from build123d import *

# Parameters (mm, degrees)
EXTRUDE_1_DEPTH          = 24
CUT_EXTRUDE_2_DEPTH      = 54.111509792
CUT_EXTRUDE_2_DEPTH_BACK = 40
CUT_EXTRUDE_START        = -40
CUT_EXTRUDE_3_DEPTH      = 40
SKETCH_8_R               = 2
SKETCH_8_R_2             = 5
CUT_EXTRUDE_4_DEPTH      = 40
SKETCH_9_R               = 1.5
CUT_EXTRUDE_5_DEPTH      = 10


with BuildPart() as part:
    # 草图1 → 凸台-拉伸1 (new body)
    with BuildSketch(Plane.XY):
        with BuildLine():
            Line((30, -7), (30, -34))
            Line((30, -34), (32.997461605, -34))
            Line((32.997461605, -34), (32.997461605, -3))
            ThreePointArc((32.997461605, -3), (32.118781948, -0.878679656), (29.997461605, 0))
            Line((29.997461605, 0), (0, 0))
            Line((0, 0), (0, -4))
            Line((0, -4), (27, -4))
            ThreePointArc((27, -4), (29.121320344, -4.878679656), (30, -7))
        make_face()
    extrude(amount=EXTRUDE_1_DEPTH)

    # 草图4 → 切除-拉伸2 (cut, two sides: drawn at the far end of the back side and taken through both)
    with BuildSketch(Plane(origin=(32.997461605, 0, 0), x_dir=(0, 0, -1), z_dir=(1, 0, 0)).offset(-CUT_EXTRUDE_2_DEPTH_BACK)):
        with BuildLine():
            Line((-24, -34), (-12, -34))
            ThreePointArc((-12, -34), (-20.485281374, -30.485281374), (-24, -22))
            Line((-24, -22), (-24, -34))
        make_face()
    extrude(amount=CUT_EXTRUDE_2_DEPTH + CUT_EXTRUDE_2_DEPTH_BACK, mode=Mode.SUBTRACT)

    # 草图7 → 切除-拉伸3 (cut)
    with BuildSketch(Plane(origin=(32.997461605, 0, 0), x_dir=(0, 0, -1), z_dir=(1, 0, 0)).offset(CUT_EXTRUDE_START)):
        with BuildLine():
            Line((0, -34), (0, -22))
            ThreePointArc((0, -22), (-3.514718626, -30.485281374), (-12, -34))
            Line((-12, -34), (0, -34))
        make_face()
    extrude(amount=CUT_EXTRUDE_3_DEPTH, mode=Mode.SUBTRACT)

    # 草图8 → 切除-拉伸4 (cut)
    with BuildSketch(Plane(origin=(0, 0, 0), x_dir=(1, 0, 0), z_dir=(0, 1, 0))):
        with Locations(Location((7.95757976, -5.000064267, 0), (0, 0, 270))):
            Circle(SKETCH_8_R)
        with Locations(Location((22, -19, 0), (0, 0, 270))):
            Circle(SKETCH_8_R)
        with Locations(Location((21.95757976, -5.000064267, 0), (0, 0, 270))):
            Circle(SKETCH_8_R)
        with Locations(Location((15, -12, 0), (0, 0, 270))):
            Circle(SKETCH_8_R_2)
        with Locations(Location((8, -19, 0), (0, 0, 270))):
            Circle(SKETCH_8_R)
    extrude(amount=-CUT_EXTRUDE_4_DEPTH, mode=Mode.SUBTRACT)

    # 草图9 → 切除-拉伸5 (cut)
    with BuildSketch(Plane(origin=(32.997461605, 0, 0), x_dir=(0, 0, -1), z_dir=(1, 0, 0))):
        with Locations((-12.027919591, -22.255700116)):
            Circle(SKETCH_9_R)
    extrude(amount=-CUT_EXTRUDE_5_DEPTH, mode=Mode.SUBTRACT)


solid = part.part
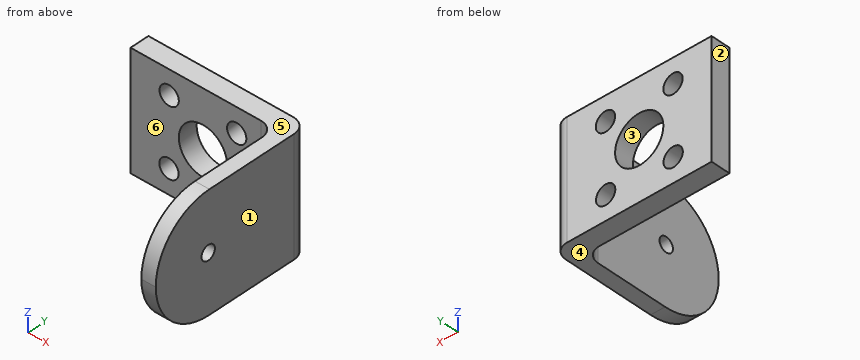
Work out the finished part from the listing and answer in its coordinate system (mm). Face numbers are marked on the shaded views. A direction names the side the tool comes from. Coordinates: 2 decimals unless noted, no trailing zeros. Loops run counter-clockwise (first coordinate to the right, second up) from the corner with the lowest first, then second, coordinate; pieces in that order, holes last. Notation, with made-up numbers: (53, -37) -> (72, -37) arc R24 ccw to (72, -14) -> close; hole circle Ø3 at (3, 6.25). An arc over 180 degrees is marked (long way). Write each question's results on one line, items separated by ' | '. Start each with the question number.
1) For the marked faces 5 and 6, determine the directions among +Z, -Z, +X, -X, +Y, -Y from which every point of the face is accessible in a straight line to the end or side of a thin tool.
2) Consider line 1 along X through (y, z) = (-1.3, 19); line 2 along Y through (x, z) = (27, 3); line 3 along X through (y, z) = (-29, 12). Determine where each line is inside the solid, lowest interval first.
3) The mould has two halves that part along X. Classify the marked faces 1, 2, 3 and 4: pulls with the +X half, pulls with the -X half, needs draft (parallel to the pull), parting line crosses it, or undercut.
4) Find section D-D on z = 22. Determine the outline of the cut face in (x, y).
5) Flat-ended cylindrical pins translate along their axes: P1, Ø2.5, axis at x = 8, z = 19, coming from the +Y side; P2, Ø12, axis at y = -19.5, z = 17, coming from the -X side; P3, Ø6.5, axis at x = 22, z = 19, coming from the -Y side; P4, Ø3, axis at y = -6.5, z = 8.5, coming from the -X side. Find the tip coordinate at first contact, or state that the pin passes through.
6) Find section C-C on y = -1.5. Determine the outline of the cut face in (x, z).
7) Find section A-A on z = 19. Determine the outline of the cut face in (x, y), then the cut area to 3 significant figures.
8) Find section B-B on x = 20.5. Determine the outline of the cut face in (y, z).
Response values:
1) face 5: +Z, +X, -X, +Y, -Y | face 6: +Z, -Z, -X, -Y
2) line 1: x = 0 to 6, 10 to 20, 24 to 32.47 | line 2: y = -4 to 0 | line 3: x = 30 to 33
3) face 1: pulls with the +X half | face 2: pulls with the -X half | face 3: undercut | face 4: needs draft
4) outline: (0, -4) -> (27, -4) arc R3 cw to (30, -7) -> (30, -28.63) -> (33, -28.63) -> (33, -3) arc R3 ccw to (30, 0) -> (0, 0) -> close
5) P1: passes through | P2: stops at x = 30 | P3: stops at y = -4 | P4: stops at x = 29.24
6) outline: (0, 0) -> (32.6, 0) -> (32.6, 24) -> (0, 24) -> close; hole circle Ø4 at (7.96, 5); hole circle Ø4 at (8, 19); hole circle Ø10 at (15, 12); hole circle Ø4 at (21.96, 5); hole circle Ø4 at (22, 19)
7) outline: (0, -4) -> (6, -4) -> (6, 0) -> (0, 0) -> close; (10, -4) -> (20, -4) -> (20, 0) -> (10, 0) -> close; (24, -4) -> (27, -4) arc R3 cw to (30, -7) -> (30, -31.75) -> (33, -31.75) -> (33, -3) arc R3 ccw to (30, 0) -> (24, 0) -> close | area: 183 mm^2
8) outline: (-4, 0) -> (0, 0) -> (0, 3.63) -> (-4, 3.63) -> close; (-4, 6.37) -> (0, 6.37) -> (0, 17.68) -> (-4, 17.68) -> close; (-4, 20.32) -> (0, 20.32) -> (0, 24) -> (-4, 24) -> close
